Job drawing, mm, ordinate dimensions from the low corner. One solid piece. A direction names the side the tool comes from. Coordinates: 2 decimals unless noted, no trailing zeros. Order: outer loops, then holes, each group sorted by start corner. A loop starts at its lowest first (then second) coordinate and runs counter-clockwise, first axis right, second up. Notation, with made-up numbers: M -35,26 L 13,26 A16 cw 13,46 Z; hole C 42,48 d6. An arc over 180 degrees is marked long. Write item = value, one per line. Start each with the question number.
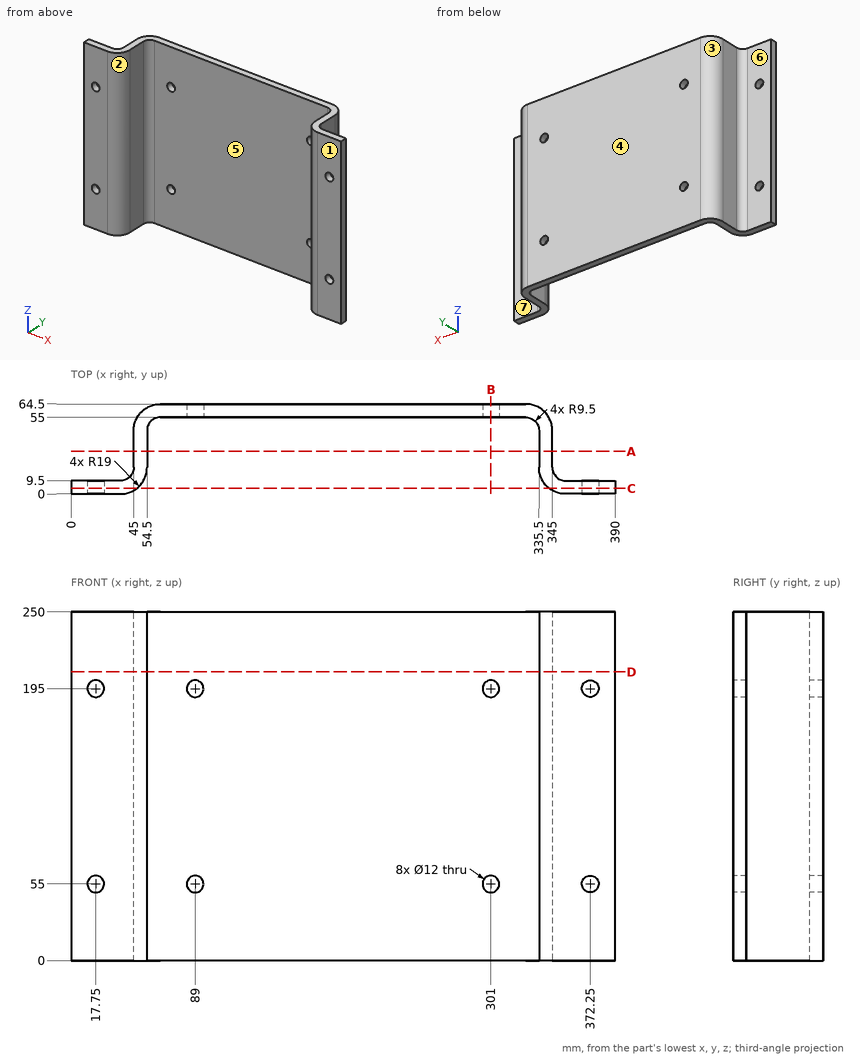
1. Slice it at D-D (z = 207). Write the cut outline in (x, y).
2. Probe L1, parallel to Z at x = 301, y = 59.75; L2, parallel to X at y = 62, z = 55; L3, parallel to X at y = 3, z = 195. List the from-to ranges inside material, lowest first.
3. Flat gauge pins, fed straight in: pin 1 (2 mm diameter, centred on x = 129.5, z = 75.5, fed in from -Y); pin 2 (15.5 mm diameter, centred on x = 372.25, z = 55, fed in from +Y); pin 3 (13 mm diameter, centred on y = 28, z = 160.5, fed in from -X); pin 4 (7 mm diameter, centred on x = 301, z = 195, fed in from +Y). Where does each tip first touch, or does it go through?
4. Mould opens along X. For the marked faces 1, 2 and 3 say: released by +X, released by -X, zero draft, split by the parting line, or undercut.
5. Slice it at A-A (y = 30.5). Write the cut outline in (x, z), plus the area to 3 significant figures.
6. 3-axis set-ups, long thin cutter, end or side, ignore diameter. For the marked faces 4, 5, 6 and 7: which of +Z, -Z, +X, -X, +Y, -Y reach the whole face in a straight line?
7. Slice it at C-C (y = 4). Write the cut outline in (x, z).
8. Slice it at B-B (x = 301). Write the cut outline in (y, z), plus the area to 3 significant figures.
Calculated:
q1.outline = M 0,0 L 35.5,0 A19 ccw 54.5,19 L 54.5,45.5 A9.5 cw 64,55 L 326,55 A9.5 cw 335.5,45.5 L 335.5,19 A19 ccw 354.5,0 L 390,0 L 390,9.5 L 354.5,9.5 A9.5 cw 345,19 L 345,45.5 A19 ccw 326,64.5 L 64,64.5 A19 ccw 45,45.5 L 45,19 A9.5 cw 35.5,9.5 L 0,9.5 Z
q2.L1 = 0 to 49, 61 to 189, 201 to 250
q2.L2 = 54.58 to 83, 95 to 295, 307 to 335.42
q2.L3 = 0 to 11.75, 23.75 to 45.75, 344.25 to 366.25, 378.25 to 390
q3.pin_1 = 55
q3.pin_2 = 9.5
q3.pin_3 = 45
q3.pin_4 = through
q4.face_1 = zero draft
q4.face_2 = undercut
q4.face_3 = released by -X
q5.outline = M 45,0 L 54.5,0 L 54.5,250 L 45,250 Z; M 335.5,0 L 345,0 L 345,250 L 335.5,250 Z
q5.area = 4,750 mm²
q6.face_4 = +Z, -Z, +X, -X, +Y
q6.face_5 = +Z, -Z, -Y
q6.face_6 = +Z, -Z, -X, +Y
q6.face_7 = +Z, -Z, +X, +Y
q7.outline = M 0,0 L 47.16,0 L 47.16,250 L 0,250 Z; M 342.84,0 L 390,0 L 390,250 L 342.84,250 Z; hole C 17.75,55 d12; hole C 17.75,195 d12; hole C 372.25,55 d12; hole C 372.25,195 d12
q8.outline = M 55,0 L 64.5,0 L 64.5,49 L 55,49 Z; M 55,61 L 64.5,61 L 64.5,189 L 55,189 Z; M 55,201 L 64.5,201 L 64.5,250 L 55,250 Z
q8.area = 2,150 mm²
